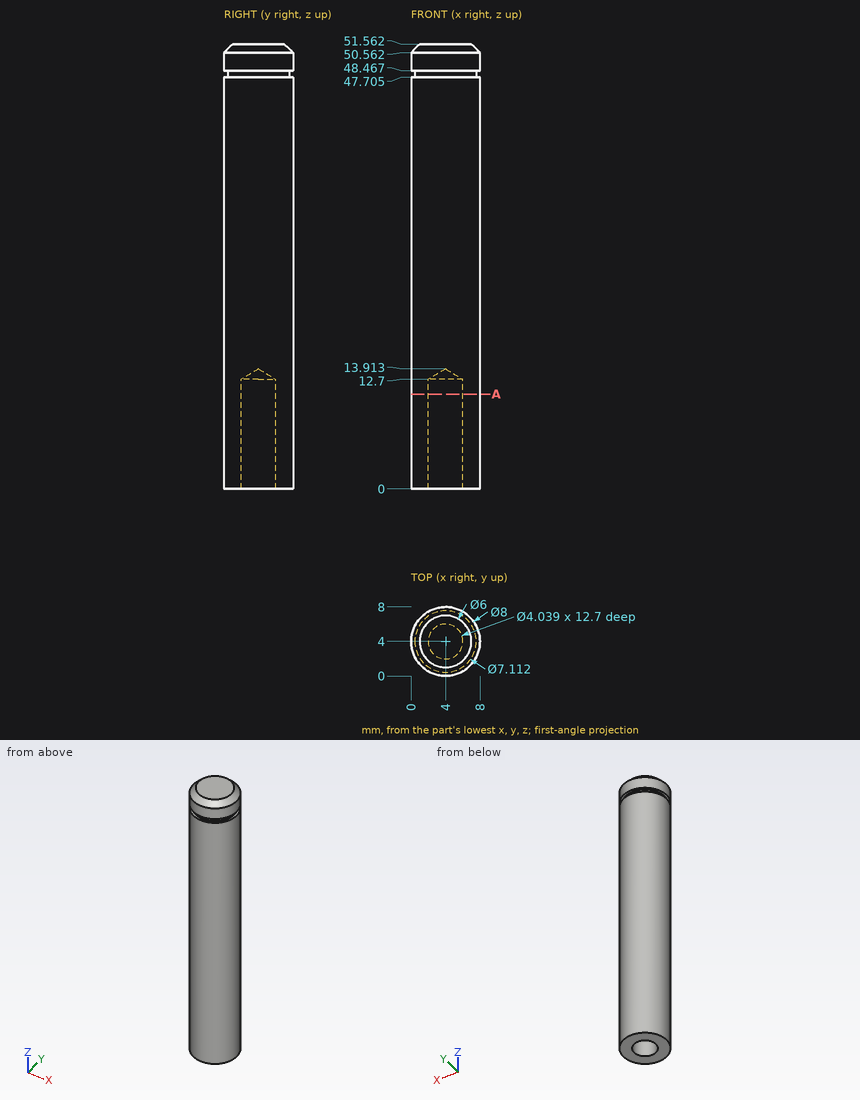
Design review of the part shown in the three views and the two pictorial views. Dimensions are in mm from the part's minimum x, y and z. Round coordinates to 2 decimals unless told otherwise and drop trailing zeros. Loops run counter-clockwise (first coordinate to the right, second up) from the corner with the lowest first, then second, coordinate; pieces in that order, holes last. Notation, with made-up numbers: (19, -3.75) -> (23, -3.75) arc R18 cw to (23, 28.25) -> close; hole circle Ø7 at (-34.5, -17). An arc over 180 degrees is marked (long way). Answer as a JSON object with one key per item and string values. Group by question number.
1) We need section A-A on z = 11. Write out the cut boundary in (x, y).
2) For pin 1 Ø3 at (y, z) = (6, 37.5) entering from +X, flat-tipped, find the tip position at first contact; note if it passes through.
3) For line 1 (X direction, y = 4, z = 3.5); line 2 (Y direction, x = 4.25, z = 38), list the stretches that pass through material, from the lowest coordinate up. Write a range as [from, to].
Result set:
{
 "1": {"outline": "circle Ø8 at (4, 4); hole circle Ø4.04 at (4, 4)"},
 "2": {"pin 1": "x = 7.97"},
 "3": {"line 1": "[0, 1.98], [6.02, 8]", "line 2": "[0.01, 7.99]"}
}
